Study the drawing (mm; zero at the part's minimum x, y, z) and answer. Round coordinates to 2 decimals unless told otherwise and drop trailing zeros. Loops run counter-clockwise (first coordinate to the right, second up) from the corner with the lowest first, then second, coordinate; pieces in that order, holes last. Notation, with made-up numbers: M 44,-16.75 L 50,-16.75 A19 ccw 50,-9.75 Z; hole C 2.5,-36.5 d9. An arc over 180 degrees is marked long. Put each result on its own line as item: value. Start each with the question number.
(1) Determine the mould class of the marked faces 1, 2 and 3 for opening direction X: released by +X, released by -X, zero draft, split by the parting line, or undercut.
(2) Section A-A, the plane x = 50.8 is taken. Determine the outline of the cut face in (y, z).
(3) Section B-B, the plane y = 13.25 is taken. Determine the outline of the cut face in (x, z), then the cut area to 3 significant figures.
(4) Straight lines are drawn through the part: line 1 (Z direction, x = 50.8, y = 18.25); line 2 (X direction, y = 9.5, z = 56); line 3 (Z direction, x = 78, y = 5.75). For each, find the intervals that lie inside material, in ascending order.
(5) Flat-ended cylindrical pins translate along their axes: P1, Ø4, axis at y = 12, z = 10.5, coming from the +X side; P2, Ø4, axis at y = 12.5, z = 34.5, coming from the -X side; P3, Ø4, axis at y = 3.5, z = 25.5, coming from the -X side; P4, Ø10, axis at x = 50.8, z = 50.8, coming from the +Y side. Find the tip coordinate at first contact, or state that the pin passes through.
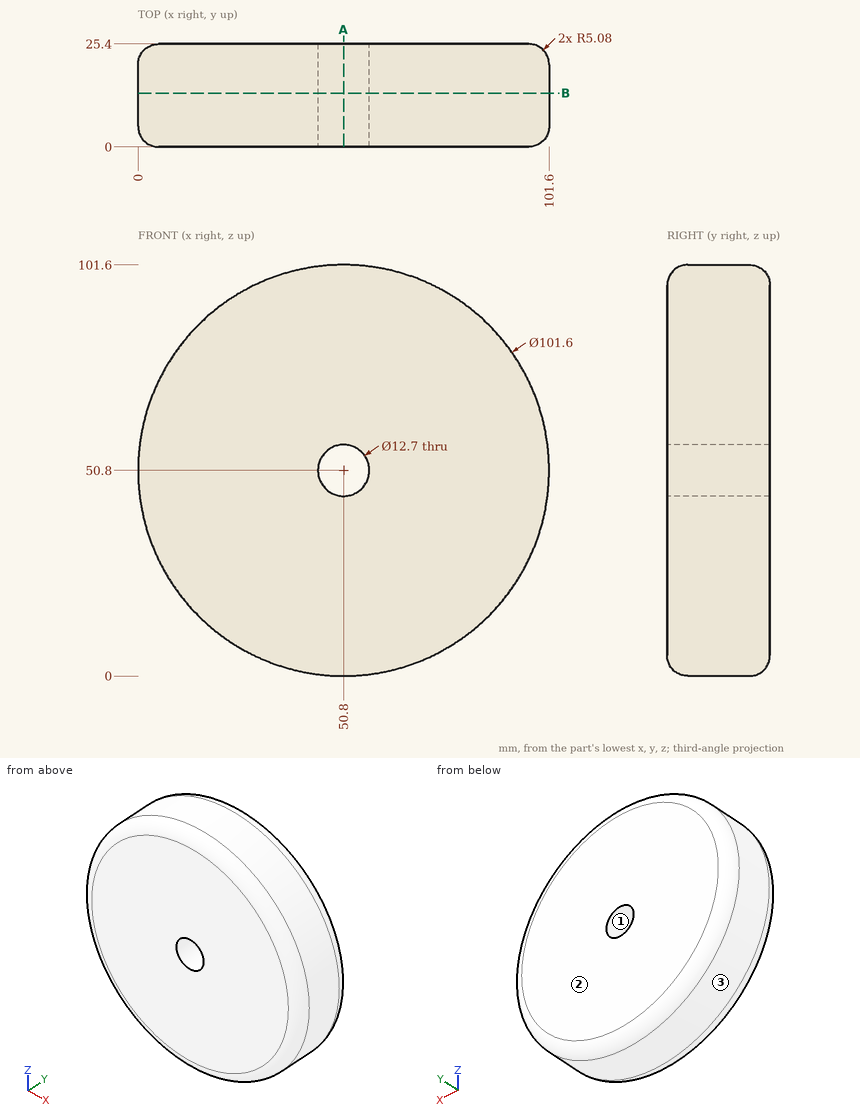
Recorded:
1. face 1: undercut
1. face 2: zero draft
1. face 3: split by the parting line
2. outline: M 0,5.08 A5.08 ccw 5.08,0 L 20.32,0 A5.08 ccw 25.4,5.08 L 25.4,44.45 L 0,44.45 Z; M 0,57.15 L 25.4,57.15 L 25.4,96.52 A5.08 ccw 20.32,101.6 L 5.08,101.6 A5.08 ccw 0,96.52 Z
3. outline: C 50.8,50.8 d101.6; hole C 50.8,50.8 d12.7
3. area: 7,980 mm²
4. line 1: z = 0 to 44.45, 57.15 to 101.6
4. line 2: x = 0.27 to 47.16, 54.44 to 101.33
4. line 3: z = 7.9 to 93.7
5. P1: stops at x = 84.17
5. P2: stops at x = 2.05
5. P3: stops at x = 5.81
5. P4: passes through
